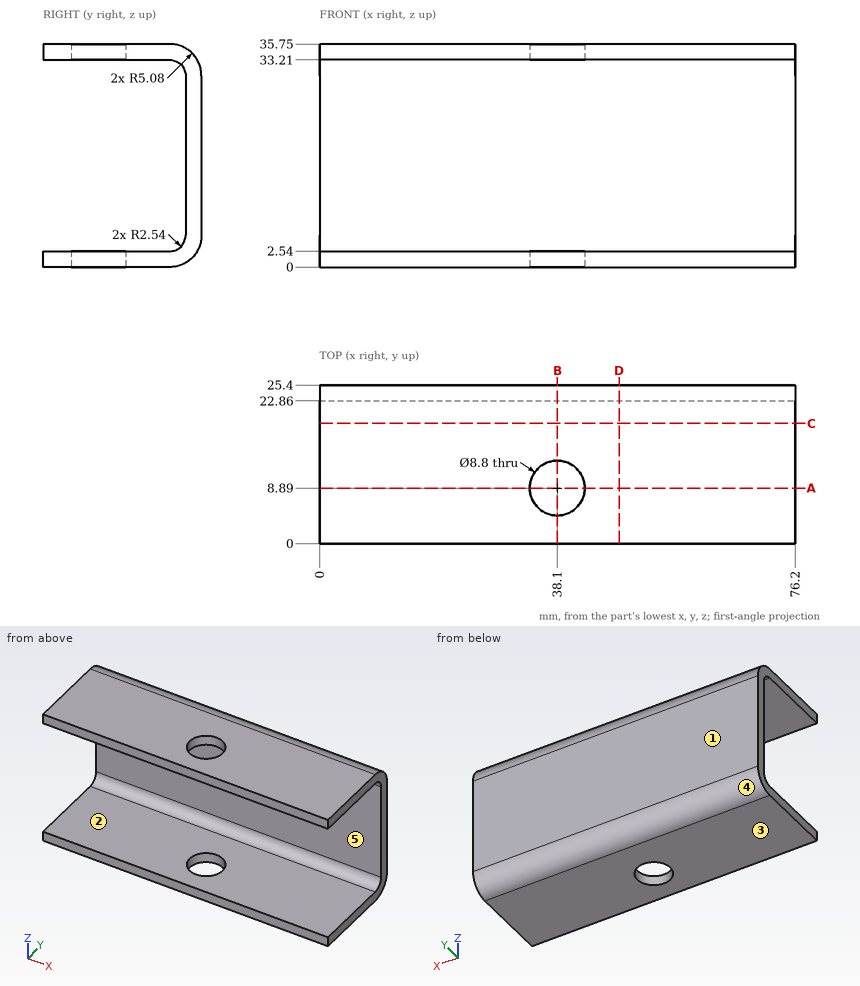
Input: dimensioned drawing with shaded views. Units: mm. Origin: part minimum x, y, z. A direction names the side the tool comes from. Round coordinates to 2 decimals unless told otherwise and drop trailing zeros. Order: outer loops, then holes, each group sorted by start corner. A loop starts at its lowest first (then second) coordinate and runs counter-clockwise, first axis right, second up. Notation, with made-up numbers: (21.25, 37) -> (54.25, 37) arc R32 ccw to (54.25, 75) -> close; hole circle Ø2 at (-20, 35). An arc over 180 degrees is marked (long way). Put each result on its own line as item: value. Start each with the question number.
Q1. Section A-A on y = 8.89. Return the cut outline in (x, z).
Q2. Reachability of the marked faces 4 and 5 from +Z, -Z, +X, -X, +Y, -Y: full face, straight path, thin tool, end or side. Return the list, or none.
Q3. Section C-C on y = 19.25. Return the cut outline in (x, z), and give its area (3 significant figures).
Q4. Pull-direction query (Z, two-part tool) for the marked faces 1, 2 and 3; classes: +Z half, -Z half, draft (parallel to the pull), parting line (faces both ways), or undercut.
Q5. Section D-D on x = 48. Return the cut outline in (y, z), and give its area (3 significant figures).
Q6. First-contact query: pin 1 (1 mm diameter, centred on x = 44, z = 10.5, fed in from -Y). Flat tip, straight axial feed; report the tip coordinate or a pass-through.
Q7. Line query: probe 1 along X at (y, z) = (8.89, 0.85); probe 2 along Z at (x, y) = (30, 11.75); probe 3 along Y at (x, z) = (71, 9). Output: solid intervals per line, ascending.
Q8. Section B-B on x = 38.1. Return the cut outline in (y, z).
Ans:
1. outline: (0, 0) -> (33.7, 0) -> (33.7, 2.54) -> (0, 2.54) -> close; (0, 33.21) -> (33.7, 33.21) -> (33.7, 35.75) -> (0, 35.75) -> close; (42.5, 0) -> (76.2, 0) -> (76.2, 2.54) -> (42.5, 2.54) -> close; (42.5, 33.21) -> (76.2, 33.21) -> (76.2, 35.75) -> (42.5, 35.75) -> close
2. face 4: -Z, +X, -X, +Y
2. face 5: +X, -X, -Y
3. outline: (0, 0) -> (76.2, 0) -> (76.2, 2.54) -> (0, 2.54) -> close; (0, 33.21) -> (76.2, 33.21) -> (76.2, 35.75) -> (0, 35.75) -> close
3. area: 387 mm2
4. face 1: draft
4. face 2: undercut
4. face 3: -Z half
5. outline: (0, 0) -> (20.32, 0) arc R5.08 ccw to (25.4, 5.08) -> (25.4, 30.67) arc R5.08 ccw to (20.32, 35.75) -> (0, 35.75) -> (0, 33.21) -> (20.32, 33.21) arc R2.54 cw to (22.86, 30.67) -> (22.86, 5.08) arc R2.54 cw to (20.32, 2.54) -> (0, 2.54) -> close
5. area: 199 mm2
6. pin 1: stops at y = 22.86
7. probe 1: x = 0 to 33.7, 42.5 to 76.2
7. probe 2: z = 0 to 2.54, 33.21 to 35.75
7. probe 3: y = 22.86 to 25.4
8. outline: (0, 0) -> (4.49, 0) -> (4.49, 2.54) -> (0, 2.54) -> close; (0, 33.21) -> (4.49, 33.21) -> (4.49, 35.75) -> (0, 35.75) -> close; (13.29, 0) -> (20.32, 0) arc R5.08 ccw to (25.4, 5.08) -> (25.4, 30.67) arc R5.08 ccw to (20.32, 35.75) -> (13.29, 35.75) -> (13.29, 33.21) -> (20.32, 33.21) arc R2.54 cw to (22.86, 30.67) -> (22.86, 5.08) arc R2.54 cw to (20.32, 2.54) -> (13.29, 2.54) -> close
